```python
from build123d import *

# Parameters (mm, degrees)
SKETCH1_W           = 7.7
SKETCH1_H           = 35
BOSS_EXTRUDE1_DEPTH = 47
SKETCH2_R           = 11.75
SKETCH2_R_2         = 3.75
CUT_EXTRUDE1_DEPTH  = 4
SKETCH3_W           = 7.7
SKETCH3_H           = 35
BOSS_EXTRUDE2_DEPTH = 20
SKETCH4_R           = 6
CUT_EXTRUDE2_DEPTH  = 0.5
FILLET1_R           = 10


with BuildPart() as part:
    # Sketch1 → Boss-Extrude1 (new body)
    with BuildSketch(Plane.XY):
        with Locations((3.85, 17.5)):
            Rectangle(SKETCH1_W, SKETCH1_H)
    extrude(amount=-BOSS_EXTRUDE1_DEPTH)

    # Sketch2 → Cut-Extrude1 (cut)
    with BuildSketch(Plane(origin=(7.7, 0, 0), x_dir=(0, 0, -1), z_dir=(1, 0, 0))):
        with Locations(Location((23.5, 17.5, 0), (0, 0, 90))):
            Circle(SKETCH2_R)
        with Locations(Location((23.5, 24.4, 0), (0, 0, 90))):
            Circle(SKETCH2_R_2, mode=Mode.SUBTRACT)
    extrude(amount=-CUT_EXTRUDE1_DEPTH, mode=Mode.SUBTRACT)

    # Sketch3 → Boss-Extrude2 (add)
    with BuildSketch(Plane.XY):
        with Locations((3.85, 17.5)):
            Rectangle(SKETCH3_W, SKETCH3_H)
    extrude(amount=BOSS_EXTRUDE2_DEPTH)

    # Sketch4 → Cut-Extrude2 (cut)
    with BuildSketch(Plane(origin=(7.7, 0, 0), x_dir=(0, 0, -1), z_dir=(1, 0, 0))):
        with Locations(Location((-10, 17.5, 0), (0, 0, 90))):
            Circle(SKETCH4_R)
    extrude(amount=-CUT_EXTRUDE2_DEPTH, mode=Mode.SUBTRACT)

    # Fillet1
    # the kernel refuses this fillet: 10 mm, written as the material it takes off along each edge
    with BuildSketch(Plane(origin=(7.7, 17.5, 10), x_dir=(0, 1, 0), z_dir=(0, 0, -1))) as fillet1_piece_1:
        with BuildLine():
            CenterArc((9.122498999, -10), FILLET1_R, 90, 18.194872339)
            Line((6, -0.5), (5.93755002, -0.31))
            ThreePointArc((5.93755002, -0.31), (5.8, -0.25), (5.8, 0))
            Line((5.8, 0), (6, 0.2))
            Line((6, 0.2), (9.122498999, 0.2))
            Line((9.122498999, 0.2), (9.122498999, 0))
        make_face()
    revolve(axis=Axis((7.7, 17.5, 10), (1, 0, 0)), mode=Mode.SUBTRACT)


solid = part.part
```
Input: part model. Units: mm. Frame: model coordinates. A direction names the side the tool comes from. Give positions to 0.01 mm unless a question says otherwise; leave off trailing zeros. Write each loop counter-clockwise with the first axis right and the second up, starting at its lowest first coordinate (ties: lowest second). Pieces come first, ordered by that corner, then holes. Notation, with made-up numbers: (30, 71.25) - (78, 71.25) arc R17 cw to (78, 76.25) - close; hole circle Ø1 at (-21.75, 87). An arc over 180 degrees is marked (long way). Write item = value, one per line. Start each with the question number.
1) Cut plane B-B (z = -23.5). Return loops of the section in (x, y), and give its area (4 significant figures).
2) Cut plane A-A (x = 6). Return loops of the section in (y, z), and give its area (3 significant figures).
3) Reachability of faces 1 (the face through (5.728, 26.13, -26.827)), 2 (the face through (0, 17, -14)) from +Z, -Z, +X, -X, +Y, -Y: full face, straight path, thin tool, end or side. Return the list, or none.
4) Material intervals for L1, parallel to X at y = 8, z = -20.5; L2, parallel to Z at x = 5.55, y = 17.5; L3, parallel to Y at x = 6.75, z = -30, sorted ascending. Write a range as [from, to].
5) Draft query along Y for faces 3 (the face through (3.7, 17, -23)), 4 (the face through (4, 18, 20)), 5 (the face through (4, 35, -14)). Return one class per face: pulls with the +Y half, pulls with the -Y half, needs draft (parallel to the pull), parting line crosses it, or undercut.
6) Pin query (flat end, axial travel): pin 1 (6 mm diameter, centred on y = 18.5, z = 11, fed in from +X). Return the tip coordinate at first contact, or that it passes through.
Answers follow:
q1.outline = (0, 0) - (7.7, 0) - (7.7, 5.75) - (3.7, 5.75) - (3.7, 20.65) - (7.7, 20.65) - (7.7, 28.15) - (3.7, 28.15) - (3.7, 29.25) - (7.7, 29.25) - (7.7, 35) - (0, 35) - close
q1.area = 205.5 mm^2
q2.outline = (0, -47) - (35, -47) - (35, 20) - (0, 20) - close; circle Ø7.5 at (24.4, -23.5); hole circle Ø23.5 at (17.5, -23.5)
q2.area = 1,960 mm^2
q3.face_1 = +X
q3.face_2 = +Z, -Z, -X, +Y, -Y
q4.L1 = [0, 3.7]
q4.L2 = [-47, -35.25], [-11.75, 20]
q4.L3 = [0, 7.71], [27.29, 35]
q5.face_3 = undercut
q5.face_4 = needs draft
q5.face_5 = pulls with the +Y half
q6.pin_1 = 7.2
